CAD build for the part. Positions are in the model's coordinates, mm. A direction names the side the tool comes from. Coordinates: 2 decimals unless noted, no trailing zeros. Loops run counter-clockwise (first coordinate to the right, second up) from the corner with the lowest first, then second, coordinate; pieces in that order, holes last. Notation, with made-up numbers: (60, 46.25) -> (107, 46.25) arc R21 cw to (107, 59.25) -> close; hole circle Ø10 at (50, 6). An arc over 180 degrees is marked (long way). Write each question's results on one line, items separated by ' | '.
from build123d import *

# Parameters (mm, degrees)
ESQUISSE1_W             = 80
ESQUISSE1_H             = 51.00000000000001
BOSS_EXTRU_1_DEPTH      = 1.5
ESQUISSE2_R             = 1.2500000000000047
ESQUISSE2_R_2           = 1.250000000000005
ESQUISSE2_W             = 55.00000000000001
ESQUISSE2_H             = 17
ENL_V_MAT_EXTRU_1_DEPTH = 65.83247642964135
CONG_1_R                = 4


with BuildPart() as part:
    # Esquisse1 → Boss.-Extru.1 (new body)
    with BuildSketch(Plane(origin=(0, 0, 0), x_dir=(1, 0, 0), z_dir=(0, 1, 0))):
        with Locations((0, -25.500000000000004)):
            Rectangle(ESQUISSE1_W, ESQUISSE1_H)
    extrude(amount=BOSS_EXTRU_1_DEPTH)

    # Esquisse2 → Enlèv. mat.-Extru.1 (cut, through all)
    with BuildSketch(Plane(origin=(0, 1.5, 0), x_dir=(1, 0, 0), z_dir=(0, 1, 0))):
        with Locations(Location((-37.5, -32.00000000000001, 0), (0, 0, 270))):
            Circle(ESQUISSE2_R)
        with Locations(Location((-37.5, -7.000000000000006, 0), (0, 0, 270))):
            Circle(ESQUISSE2_R_2)
        with Locations(Location((37.5, -7.000000000000006, 0), (0, 0, 90))):
            Circle(ESQUISSE2_R_2)
        with Locations(Location((37.5, -32.00000000000001, 0), (0, 0, 90))):
            Circle(ESQUISSE2_R)
        with Locations((0, -42.49999999999999)):
            Rectangle(ESQUISSE2_W, ESQUISSE2_H)
        with BuildLine():
            Line((-36.00000000000001, -1.029e-14), (-29.000000000000004, -9.31e-15))
            ThreePointArc((-29.000000000000004, -9.31e-15), (-32.5, -3.5000000000000115), (-36.00000000000001, -1.029e-14))
        make_face()
    extrude(amount=-ENL_V_MAT_EXTRU_1_DEPTH, mode=Mode.SUBTRACT)

    # Congé1
    # the kernel refuses this fillet: 4 mm, written as the material it adds along each edge
    with BuildSketch(Plane(origin=(-27.5, 1.5, 33.99999999999999), x_dir=(0, 0, 1), z_dir=(0, -1, 0))) as cong_1_piece_1:
        with BuildLine():
            CenterArc((CONG_1_R, -CONG_1_R), CONG_1_R, 90, 90)
            Line((0, -CONG_1_R), (0, 0))
            Line((0, 0), (CONG_1_R, 0))
        make_face()
    extrude(amount=1.5)
    with BuildSketch(Plane(origin=(27.5, 1.5, 33.99999999999999), x_dir=(0, 0, 1), z_dir=(0, -1, 0))) as cong_1_piece_2:
        with BuildLine():
            CenterArc((CONG_1_R, CONG_1_R), CONG_1_R, 180, 90)
            Line((0, CONG_1_R), (0, 0))
            Line((0, 0), (CONG_1_R, 0))
        make_face()
    extrude(amount=1.5)
    # the kernel refuses this fillet: 4 mm, written as the material it takes off along each edge
    with BuildSketch(Plane(origin=(-27.5, 11.5, 51), x_dir=(-1, 0, 0), z_dir=(0, -1, 0)), Plane(origin=(40, -10, 51), x_dir=(0, 0, -1), z_dir=(0, 1, 0)), Plane(origin=(-40, -10, 51), x_dir=(1, 0, 0), z_dir=(0, 1, 0))) as cong_1_2_piece_1:
        with BuildLine():
            CenterArc((CONG_1_R, CONG_1_R), CONG_1_R, 180, 90)
            Line((0, CONG_1_R), (0, 0))
            Line((0, 0), (CONG_1_R, 0))
        make_face()
    extrude(amount=21.5, mode=Mode.SUBTRACT)
    with BuildSketch(Plane(origin=(27.5, 11.5, 51), x_dir=(1, 0, 0), z_dir=(0, -1, 0))) as cong_1_2_piece_2:
        with BuildLine():
            CenterArc((CONG_1_R, -CONG_1_R), CONG_1_R, 90, 90)
            Line((0, -CONG_1_R), (0, 0))
            Line((0, 0), (CONG_1_R, 0))
        make_face()
    extrude(amount=21.5, mode=Mode.SUBTRACT)
    with BuildSketch(Plane(origin=(-29, 8.610721925562018, 0), x_dir=(-0.27757416183489847, 0, 0.9607042128988784), z_dir=(0, -1, 0))) as cong_1_2_piece_3:
        with BuildLine():
            CenterArc((3.0533157801839375, -3.842816851595507), CONG_1_R, 106.11547631775109, 57.76904736449852)
            Line((-0.7895010714115829, -2.732520204255937), (0, 0))
            ThreePointArc((0, 0), (0.9715095664221598, -0.13753525485392898), (1.9430191328443203, 7e-17))
        make_face()
    extrude(amount=15.721443851124036, mode=Mode.SUBTRACT)
    with BuildSketch(Plane(origin=(-36, 8.610721925562018, 0), x_dir=(-1, 0, 0), z_dir=(0, -1, 0))) as cong_1_2_piece_4:
        with BuildLine():
            CenterArc((2.844288770224807, -4), CONG_1_R, 90, 57.769047364498164)
            ThreePointArc((-0.5393319072284086, -1.8666666666666827), (-0.1375352548539297, -0.9715095664221669), (0, 0))
            Line((0, 0), (2.844288770224807, 0))
        make_face()
    extrude(amount=15.721443851124036, mode=Mode.SUBTRACT)
    with BuildSketch(Plane(origin=(-40, -10, 0), x_dir=(0, 0, 1), z_dir=(0, 1, 0))) as cong_1_2_piece_5:
        with BuildLine():
            CenterArc((CONG_1_R, CONG_1_R), CONG_1_R, 180, 90)
            Line((-4.4e-16, CONG_1_R), (0, 0))
            Line((0, 0), (CONG_1_R, 0))
        make_face()
    extrude(amount=21.5, mode=Mode.SUBTRACT)
    with BuildSketch(Plane(origin=(40, -10, 0), x_dir=(-1, 0, 0), z_dir=(0, 1, 0))) as cong_1_2_piece_6:
        with BuildLine():
            CenterArc((CONG_1_R, CONG_1_R), CONG_1_R, 180, 90)
            Line((0, CONG_1_R), (0, 0))
            Line((0, 0), (CONG_1_R, 0))
        make_face()
    extrude(amount=21.5, mode=Mode.SUBTRACT)


solid = part.part
1) Two-plate mould, pull along X, no slides. Class faces 1 (the flat face through (-40, 1, 26)), 2 (the cylindrical face through (38.859, 0.739, 1.203)), 3 (the cylindrical face through (28.703, 0.761, 49.859)): pulls with the +X half, pulls with the -X half, needs draft (parallel to the pull), parting line crosses it, or undercut.
Outcome:
face 1: pulls with the -X half | face 2: pulls with the +X half | face 3: undercut
2) Slice it at C-C (x = 37.5). Write the cut outline in (y, z), then the cut area to 3 significant figures.
Outcome:
outline: (0, 0.29) -> (1.5, 0.29) -> (1.5, 5.75) -> (0, 5.75) -> close; (0, 8.25) -> (1.5, 8.25) -> (1.5, 30.75) -> (0, 30.75) -> close; (0, 33.25) -> (1.5, 33.25) -> (1.5, 50.71) -> (0, 50.71) -> close | area: 68.1 mm^2
3) Slice it at A-A (z = 7). Write the cut outline in (x, y), then the cut area to 4 significant figures.
Outcome:
outline: (-40, 0) -> (-38.75, 0) -> (-38.75, 1.5) -> (-40, 1.5) -> close; (-36.25, 0) -> (36.25, 0) -> (36.25, 1.5) -> (-36.25, 1.5) -> close; (38.75, 0) -> (40, 0) -> (40, 1.5) -> (38.75, 1.5) -> close | area: 112.5 mm^2
4) Slice it at B-B (y = 0.5). Write the cut outline in (x, z), then the cut area to 3 significant figures.
Outcome:
outline: (-40, 4) arc R4 ccw to (-37.42, 0.26) arc R4 ccw to (-35.46, 1.87) arc R3.5 cw to (-29.54, 1.87) arc R4 ccw to (-26.16, 0) -> (36, 0) arc R4 ccw to (40, 4) -> (40, 47) arc R4 ccw to (36, 51) -> (31.5, 51) arc R4 ccw to (27.5, 47) -> (27.5, 38) arc R4 cw to (23.5, 34) -> (-23.5, 34) arc R4 cw to (-27.5, 38) -> (-27.5, 47) arc R4 ccw to (-31.5, 51) -> (-36, 51) arc R4 ccw to (-40, 47) -> close; hole circle Ø2.5 at (-37.5, 7); hole circle Ø2.5 at (-37.5, 32); hole circle Ø2.5 at (37.5, 7); hole circle Ø2.5 at (37.5, 32) | area: 3,090 mm^2
5) Which spindle directions (+Z, -Z, +X, -X, +Y, -Y) get a long thin tool onto all of the face, cutting with end or side? Do faces 4 (the flat face through (34, 1, 51)), 5 (the cylindrical face through (-36.325, 0.761, 0.893)), 6 (the flat face through (-27.5, 1, 43)). Say none if no direction does.
Outcome:
face 4: +Z, +X, -X, +Y, -Y | face 5: -Z, +Y, -Y | face 6: +Z, +Y, -Y
6) Pin check, flat tips, straight feed: pin 1 (2 mm diameter, centred on x = 37.5, z = 7, fed in from -Y); pin 2 (1 mm diameter, centred on x = -22, z = 6.5, fed in from -Y). Stop position of each tip, or through.
Outcome:
pin 1: passes through | pin 2: stops at y = 0
7) Slice it at D-D (x = -10.5). Write the cut outline in (y, z), then the cut area to 3 significant figures.
Outcome:
outline: (0, 0) -> (1.5, 0) -> (1.5, 34) -> (0, 34) -> close | area: 51.0 mm^2
8) Drill centre lines: L1, parallel to X at y = 0.85, z = 32; L2, parallel to Z at x = 37.5, y = 0.4; L3, parallel to Z at x = -19.5, y = 0.45. Where is each one in solid material? Low to high. Write a range as from..to.
Outcome:
L1: x = -40..-38.75, -36.25..36.25, 38.75..40 | L2: z = 0.29..5.75, 8.25..30.75, 33.25..50.71 | L3: z = 0..34
